Model file for the job. Use its own axes, mm. A direction names the side the tool comes from. Give positions to 0.01 mm unless a question says otherwise; leave off trailing zeros. Loops run counter-clockwise (first coordinate to the right, second up) from the corner with the lowest first, then second, coordinate; pieces in that order, holes last. Notation, with made-up numbers: M 16.5,80 L 50.5,80 A13 cw 50.5,87 Z; hole C 22,10 d1. An arc over 180 degrees is marked long. Answer in a Markdown table with one row per item.
```python
from build123d import *

# Parameters (mm, degrees)
F0_W     = 102.4136152118
F0_H     = 18.15164648
F1_DEPTH = 56.388
F2_W     = 25.0601731241
F2_H     = 34.5359966159
F3_DEPTH = 304.546
F4_R     = 15.2325553806
F5_DEPTH = 58.928
F6_R     = 15.4275535789
F7_DEPTH = 84.328


with BuildPart() as f1:
    # F0 (on Top) → F1 (new body)
    with BuildSketch(Plane.XY):
        with Locations((-20.018090494, 37.0683530346)):
            Rectangle(F0_W, F0_H)
        Polygon((-71.2248980999, 27.9925297946), (-71.2248980999, 46.1441762745), (-140.0751024485, 38.4146161377), (-163.9562547207, 18.7738258392), (-153.9280861616, -54.3515346944), (-133.5243433714, -54.3515346944), (-114.2685189843, 27.9925297946), align=None)
    extrude(amount=F1_DEPTH)

    # F2 (on face) → F3 (join)
    with BuildSketch(Plane.XZ.offset(-27.9925297946)):
        with Locations((-46.5627107769, 17.2679983079)):
            Rectangle(F2_W, F2_H)
    extrude(amount=F3_DEPTH)

    # F4 (on face) → F5 (join)
    with BuildSketch(Plane.YZ.offset(31.1887171119)):
        with Locations((35.7915498316, 32.1561060846)):
            Circle(F4_R)
    extrude(amount=F5_DEPTH)

    # F6 (on face) → F7 (join)
    with BuildSketch(Plane.YZ.offset(90.1167171119)):
        with Locations((35.7915498316, 32.1561060846)):
            Circle(F6_R)
    extrude(amount=F7_DEPTH)


solid = f1.part
```
Q1. Drop flat-ended pins along their axis: pin 1 (3 mm diameter, centred on x = 3.5, z = 43, fed in from +Y); pin 2 (17.5 mm diameter, centred on y = -130.5, z = 16, fed in from +X); pin 3 (9.5 mm diameter, centred on y = 35.5, z = 29, fed in from -X); pin 4 (2 mm diameter, centred on y = -74, z = 36, fed in from -X). Give the stop position or say it passes through.
Reported:
| item | result |
|---|---|
| pin 1 | y = 46.14 |
| pin 2 | x = -34.03 |
| pin 3 | x = -149.39 |
| pin 4 | through |
Q2. Saw through at A-A (z = 6). Give the cut face in (x, y).
Reported:
| item | result |
|---|---|
| outline | M -163.96,18.77 L -153.93,-54.35 L -133.52,-54.35 L -114.27,27.99 L -59.09,27.99 L -59.09,-276.55 L -34.03,-276.55 L -34.03,27.99 L 31.19,27.99 L 31.19,46.14 L -71.22,46.14 L -140.08,38.41 Z |
Q3. Saw through at B-B (y = -39). Give the cut face in (x, z), and give its area (3 significant figures).
Reported:
| item | result |
|---|---|
| outline | M -156.03,0 L -129.93,0 L -129.93,56.39 L -156.03,56.39 Z; M -59.09,0 L -34.03,0 L -34.03,34.54 L -59.09,34.54 Z |
| area | 2,340 mm² |
Q4. Saw through at D-D (y = -229.5). Give the cut face in (x, z), and give its area (3 significant figures).
Reported:
| item | result |
|---|---|
| outline | M -59.09,0 L -34.03,0 L -34.03,34.54 L -59.09,34.54 Z |
| area | 865 mm² |
Q5. Probe probe 1 along X at (y, z) = (26, 26); probe 2 along X at (y, z) = (-241, 22); probe 3 along Z at (x, y) = (145.5, 36). List the from-to ranges inside material, lowest first.
Reported:
| item | result |
|---|---|
| probe 1 | -155.17 to -114.73, -59.09 to -34.03, 31.19 to 174.44 |
| probe 2 | -59.09 to -34.03 |
| probe 3 | 16.73 to 47.58 |
Q6. Mould opens along X. For faces 1 (the face through (131.69, 23.55, 22.77)), 2 (the face through (-159.01, -17.28, 27.8)), 3 (the face through (-43, 27.993, 40)) say: released by +X, released by -X, zero draft, split by the parting line, or undercut.
Reported:
| item | result |
|---|---|
| face 1 | zero draft |
| face 2 | released by -X |
| face 3 | undercut |
Q7. 3-axis set-ups, long thin cutter, end or side, ignore diameter. For faces 4 (the face through (-144, -54.352, 28)), 5 (the face through (-52, -55, 0)), 6 (the face through (-59.093, -122, 17)): which of +Z, -Z, +X, -X, +Y, -Y reach the whole face in a straight line?
Reported:
| item | result |
|---|---|
| face 4 | +Z, -Z, -X, -Y |
| face 5 | -Z, +X, -X, +Y, -Y |
| face 6 | +Z, -Z, -Y |
Q8. Saw through at C-C (x = -46). Give the cut face in (y, z), and give its area (3 significant figures).
Reported:
| item | result |
|---|---|
| outline | M -276.55,0 L 46.14,0 L 46.14,56.39 L 27.99,56.39 L 27.99,34.54 L -276.55,34.54 Z |
| area | 11,500 mm² |
